from build123d import *

# Parameters (mm, degrees)
SKETCH1_R           = 2.15
SKETCH1_R_2         = 6.15
SKETCH1_R_3         = 1.75
SKETCH1_R_4         = 1.4
SKETCH1_W           = 7.3
SKETCH1_H           = 3.2
BOSS_EXTRUDE1_DEPTH = 4.55
SKETCH2_W           = 30.597245163
SKETCH2_H           = 76.240319195
CUT_EXTRUDE1_DEPTH  = 5.55


with BuildPart() as part:
    # Sketch1 → Boss-Extrude1 (new body)
    with BuildSketch(Plane(origin=(0, 0, 0), x_dir=(1, 0, 0), z_dir=(0, 1, 0))):
        with BuildLine():
            Line((5, 0), (83.06, 0))
            ThreePointArc((83.06, 0), (86.595533906, 1.464466094), (88.06, 5))
            Line((88.06, 5), (88.06, 10.2))
            Line((88.06, 10.2), (109.36, 10.2))
            ThreePointArc((109.36, 10.2), (112.895533906, 11.664466094), (114.36, 15.2))
            Line((114.36, 15.2), (114.36, 64.57))
            ThreePointArc((114.36, 64.57), (112.895533906, 68.105533906), (109.36, 69.57))
            Line((109.36, 69.57), (88.06, 69.57))
            Line((88.06, 69.57), (88.06, 69.73))
            ThreePointArc((88.06, 69.73), (86.595533906, 73.265533906), (83.06, 74.73))
            Line((83.06, 74.73), (5, 74.73))
            ThreePointArc((5, 74.73), (1.464466094, 73.265533906), (0, 69.73))
            Line((0, 69.73), (0, 5))
            ThreePointArc((0, 5), (1.464466094, 1.464466094), (5, 0))
        make_face()
        with Locations((5.15, 59.83)):
            Circle(SKETCH1_R, mode=Mode.SUBTRACT)
        with Locations((33.35, 59.83)):
            Circle(SKETCH1_R, mode=Mode.SUBTRACT)
        with Locations((52.45, 59.83)):
            Circle(SKETCH1_R, mode=Mode.SUBTRACT)
        with Locations((80.65, 59.83)):
            Circle(SKETCH1_R, mode=Mode.SUBTRACT)
        with Locations((5.15, 27.83)):
            Circle(SKETCH1_R, mode=Mode.SUBTRACT)
        with Locations((33.35, 27.83)):
            Circle(SKETCH1_R, mode=Mode.SUBTRACT)
        with Locations((52.45, 27.83)):
            Circle(SKETCH1_R, mode=Mode.SUBTRACT)
        with Locations((80.65, 27.83)):
            Circle(SKETCH1_R, mode=Mode.SUBTRACT)
        with Locations((94.47, 39.69)):
            Circle(SKETCH1_R_2, mode=Mode.SUBTRACT)
        with Locations((94.45, 65.33)):
            Circle(SKETCH1_R_3, mode=Mode.SUBTRACT)
        with Locations((94.45, 15.69)):
            Circle(SKETCH1_R_3, mode=Mode.SUBTRACT)
        with Locations((63.06, 4.8)):
            Circle(SKETCH1_R_4, mode=Mode.SUBTRACT)
        with Locations((72.86, 4.8)):
            Circle(SKETCH1_R_4, mode=Mode.SUBTRACT)
        with Locations((42.45, 70.13)):
            Rectangle(SKETCH1_W, SKETCH1_H, mode=Mode.SUBTRACT)
        with Locations((42.45, 9.4)):
            Rectangle(SKETCH1_W, SKETCH1_H, mode=Mode.SUBTRACT)
    extrude(amount=BOSS_EXTRUDE1_DEPTH)

    # Sketch2 → Cut-Extrude1 (cut, through all)
    with BuildSketch(Plane(origin=(0, 4.55, 0), x_dir=(1, 0, 0), z_dir=(0, 1, 0))):
        with Locations((114.748622582, 38.120159597)):
            Rectangle(SKETCH2_W, SKETCH2_H)
    extrude(amount=-CUT_EXTRUDE1_DEPTH, mode=Mode.SUBTRACT)


solid = part.part
Could you check a few things on this model? Use its own coordinates, in mm. A direction names the side the tool comes from. Coordinates: 2 decimals unless noted, no trailing zeros. Write each loop counter-clockwise with the first axis right and the second up, starting at its lowest first coordinate (ties: lowest second). Pieces come first, ordered by that corner, then holes. Notation, with made-up numbers: (-36.75, -35) - (-20.75, -35) arc R30 cw to (-20.75, 3) - close; hole circle Ø8 at (-6, 74). An arc over 180 degrees is marked (long way). Put each result on its own line as item: value. Start each with the question number.
Q1. Thinking about a two-plate mould opening in Z: for faces 4 (the flat face through (49, 0, -38)), 5 (the cylindrical face through (86.56, 2.24, -1.43)), 6 (the flat face through (42, 2, -71.73)), which applies, pulls with the +Z half, pulls with the -Z half, needs draft (parallel to the pull), parting line crosses it, or undercut?
Q2. Which directions (+Z, -Z, +X, -X, +Y, -Y) give clear straight access to the entire face, cutting with the end or side of a thin tool? Please do faces 1 (the cylindrical face through (1, 2, -2)), 2 (the flat face through (94, 2, -69.57)), 3 (the flat face through (46.1, 2, -70)).
Q3. I want a section at A-A on z = -65.33. Write out the boundary of the cut face in (x, y), plus the area to 3 significant figures.
Q4. I want a section at C-C on x = 63.06. Write out the boundary of the cut face in (y, z).
Q5. I want a section at D-D on y = 2.3. Count the separate pieces of the cut face and the enclosed holes in it, plus the area to 3 significant figures.
Q6. Please list where these lines run through material, in increasing order: L1, parallel to X at y = 3.5, z = -27.83; L2, parallel to Z at x = 43, y = 1.4; L3, parallel to Z at x = 33.35, y = 2.65.
Q7. I'm going to push flat-ended pins straight in: P1, Ø7, axis at x = 5.15, z = -27.83, coming from the +Y side; P2, Ø1.4, axis at x = 95.5, y = 1.5, coming from the +Z side. Where does each tip first touch, or does it pass through?
Q8. I want a section at B-B on x = 45. Write out the boundary of the cut face in (y, z).
Checks:
1. face 4: needs draft
1. face 5: pulls with the +Z half
1. face 6: undercut
2. face 1: +Z, -X, +Y, -Y
2. face 2: -Z, +X, +Y, -Y
2. face 3: +Y, -Y
3. outline: (0, 0) - (92.7, 0) - (92.7, 4.55) - (0, 4.55) - close; (96.2, 0) - (99.45, 0) - (99.45, 4.55) - (96.2, 4.55) - close
3. area: 437 mm²
4. outline: (0, -74.73) - (4.55, -74.73) - (4.55, -6.2) - (0, -6.2) - close; (0, -3.4) - (4.55, -3.4) - (4.55, 0) - (0, 0) - close
5. separate pieces: 1
5. enclosed holes: 14
5. area: 6,930 mm²
6. L1: 0 to 3, 7.3 to 31.2, 35.5 to 50.3, 54.6 to 78.5, 82.8 to 99.45
6. L2: -74.73 to -71.73, -68.53 to -11, -7.8 to 0
6. L3: -74.73 to -61.98, -57.68 to -29.98, -25.68 to 0
7. P1: y = 4.55
7. P2: z = -10.2
8. outline: (0, -74.73) - (4.55, -74.73) - (4.55, -71.73) - (0, -71.73) - close; (0, -68.53) - (4.55, -68.53) - (4.55, -11) - (0, -11) - close; (0, -7.8) - (4.55, -7.8) - (4.55, 0) - (0, 0) - close
